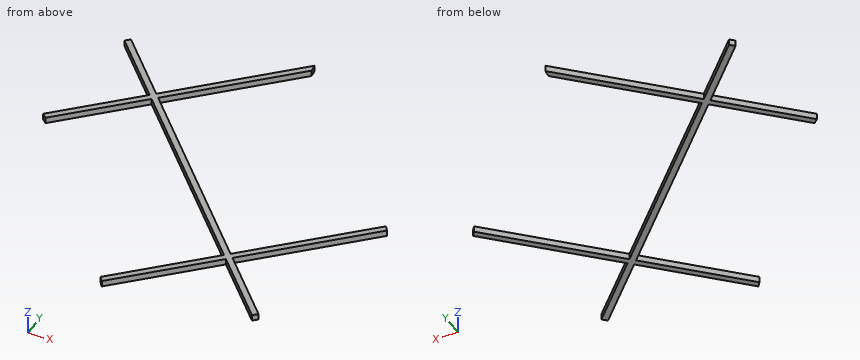
Autodesk Inventor part; units mm, degrees
ref_plane "YZ Plane" through (0, 0, 0) normal (1, 0, 0) x (0, 1, 0)
ref_plane "XZ Plane" through (0, 0, 0) normal (0, 1, 0) x (-1, 0, 0)
ref_plane "XY Plane" through (0, 0, 0) normal (0, 0, 1) x (1, 0, 0)
sketch "Sketch1" plane through (0, 0, 0) normal (0, 0, 1) x (1, 0, 0)
  arc A0 (5.5811, -56.8606) -> (20.209, -64.6836) centre (38.8796, -12.1848) ccw
  arc A1 (-7.6539, -43.4667) -> (5.5811, -56.8606) centre (37.8873, -11.7018) ccw
  arc A2 (-7.6539, -43.4667) -> (-31.2183, -12.0793) centre (-386.265, -303.1724) ccw
  arc A3 (-31.2183, -12.0793) -> (-63.3277, 19.0744) centre (-191.6112, -145.2692) ccw
  arc A4 (-67.5206, 26.3221) -> (-63.3277, 19.0744) centre (-54.6162, 28.9507) ccw
  arc A5 (-66.9469, 41.0059) -> (-67.5206, 26.3221) centre (-15.6776, 31.6496) ccw
  line L0 (-66.9469, 41.0059) -> (-26.0985, 81.0785)
  arc A6 (-3.6955, 79.7027) -> (-26.0985, 81.0785) centre (-17.6076, 36.2535) ccw
  arc A7 (1.4491, 74.6716) -> (-3.6955, 79.7027) centre (-6.1453, 72.0517) ccw
  arc A8 (2.6831, 69.1533) -> (1.4491, 74.6716) centre (-18.5892, 67.2935) ccw
  arc A9 (2.6831, 69.1533) -> (3.1898, 63.5624) centre (229.5421, 86.8959) ccw
  arc A10 (3.1898, 63.5624) -> (8.7161, 49.818) centre (30.4167, 66.5265) ccw
  arc A11 (8.7161, 49.818) -> (19.0471, 39.3259) centre (47.1297, 77.3097) ccw
  arc A12 (19.0471, 39.3259) -> (32.6891, 29.8296) centre (104.4845, 147.5139) ccw
  arc A13 (32.6891, 29.8296) -> (50.5655, 19.6706) centre (502.3948, 835.5524) ccw
  arc A14 (57.8671, 12.5741) -> (50.5655, 19.6706) centre (33.0101, -5.6965) ccw
  arc A15 (67.0572, -4.125) -> (57.8671, 12.5741) centre (18.4686, -19.9867) ccw
  arc A16 (68.9532, -23.0115) -> (67.0572, -4.125) centre (24.8632, -17.8992) ccw
  line L1 (-52.1723, 55.4999) -> (42.0363, -41.3708)
  line L2 (43.4701, -39.9764) -> (-50.7446, 56.9005)
  line L3 (42.0363, -41.3708) -> (43.4701, -39.9764)
  line L4 (-4.2615, -47.8472) -> (57.8671, 12.5741)
  line L5 (56.6239, 14.1548) -> (-5.54, -46.3007)
  line L6 (-55.2456, 12.4327) -> (2.7113, 68.7969)
  line L7 (2.3899, 71.2742) -> (-56.7711, 13.739)
  point P0 (0, 0)
  point P1 (-8.2693, 4.2237)
  point P2 (-4.9861, 4.7501)
  point P3 (-66.0155, 22.3561)
  point P4 (24.203, -20.1649)
  point P5 (22.8086, -18.7311)
  point P6 (-30.7071, 36.2969)
  point P7 (-32.1015, 37.7306)
  point P8 (-33.5353, 36.3363)
  point P9 (-32.1409, 34.9025)
  point P10 (21.3749, -20.1255)
  point P11 (22.7692, -21.5593)
  dimension "d243" = 2
  dimension "d244" = 2
  dimension "d245" = 2
extrude "Extrusion11" add sketch "Sketch1" along normal blind 2 contours L5 L1 L4 A1 | L5 L2 L4 L1 | L1 L6 L2 L5 | A3 L7 L1 L6 | L4 L2 L3 L1 | L1 L7 L2 L6 | L5 A14 L4 L2 | L1 L0 L2 L7 | L2 L7 A8 A9 L6
properties part number "print007_Grundform_Guss_innen"
For this review, take the finished solid that the model builds, in its own axes (mm). Round coordinates to 2 decimals unless told otherwise and drop trailing zeros. Write each loop counter-clockwise with the first axis right and the second up, starting at its lowest first coordinate (ties: lowest second). Pieces come first, ordered by that corner, then holes. Notation, with made-up numbers: M -37.75,-15.5 L -3.75,-15.5 A18 ccw -3.75,3.5 Z; hole C 62.25,51 d8. An arc over 180 degrees is marked long. Write item = value, one per line. Start each with the question number.
(1) Clearance check with flat-ended pins moving along their axes: pin 1 Ø1 at (y, z) = (37.5, 0.5) entering from +X; pin 2 Ø12 at (x, y) = (22, -35) entering from +Z. State where each tip first meets the part, or that it passes through.
(2) We need section B-B (x = 30.5). Give the boundary of the cut face in (y, z), then the cut area to 3 significant figures.
(3) For line 1 along X through (y, z) = (14, 1.15); line 2 along X through (y, z) = (-0.5, 1.35); line 3 along X through (y, z) = (19.5, 1.3), list the stretches that pass through material, from the lowest coordinate up.
(4) We need section A-A (y = 31.5). Give the boundary of the cut face in (x, z).
(5) We need section D-D (y = 62). Give the boundary of the cut face in (x, z), then the cut area to 3 significant figures.
(6) We need section C-C (z = 1.3). Give the boundary of the cut face in (x, y), then the cut area to 3 significant figures.
Results found:
q1.pin_1 = -28.96
q1.pin_2 = through
q2.outline = M -29.51,0 L -26.64,0 L -26.64,2 L -29.51,2 Z; M -14.04,0 L -11.25,0 L -11.25,2 L -14.04,2 Z
q2.area = 11.3 mm²
q3.line_1 = -56.5 to -53.63, -11.81 to -9.02, 56.46 to 56.75
q3.line_2 = 2.29 to 5.08, 41.55 to 44.42
q3.line_3 = -50.85 to -47.98, -17.16 to -14.37
q4.outline = M -38.51,0 L -35.64,0 L -35.64,2 L -38.51,2 Z; M -28.83,0 L -26.04,0 L -26.04,2 L -28.83,2 Z
q5.outline = M -7.15,0 L -4.28,0 L -4.28,2 L -7.15,2 Z
q5.area = 5.74 mm²
q6.outline = M -56.77,13.74 A208.49 cw -55.25,12.43 L -32.14,34.9 L 21.37,-20.13 L -5.54,-46.3 A55.52 ccw -4.26,-47.85 L 22.77,-21.56 L 42.04,-41.37 L 43.47,-39.98 L 24.2,-20.16 L 57.87,12.57 A30.85 ccw 56.62,14.15 L 22.81,-18.73 L -30.71,36.3 L 2.71,68.8 A227.7 cw 2.68,69.15 A21.35 ccw 2.39,71.27 L -32.1,37.73 L -50.74,56.9 L -52.17,55.5 L -33.54,36.34 Z
q6.area = 599 mm²
